```python
from build123d import *

# Parameters (mm, degrees)
F0_W     = 42
F0_H     = 22
F1_DEPTH = 13
F2_W     = 42
F2_H     = 22
F3_DEPTH = 5
F4_R     = 1
F5_DEPTH = 6
F6_R     = 5


with BuildPart() as f1:
    # F0 (on Top) → F1 (new body)
    with BuildSketch(Plane.XY):
        Rectangle(F0_W, F0_H)
        with BuildLine():
            ThreePointArc((-2.120368, -5.306732), (-19.5, 0), (-2.120368, 5.306732))
            Line((-2.120368, 5.306732), (2.120368, 5.306732))
            ThreePointArc((2.120368, 5.306732), (12.774302, 9.085882), (19.5, 0))
            ThreePointArc((19.5, 0), (12.774302, -9.085882), (2.120368, -5.306732))
            Line((2.120368, -5.306732), (-2.120368, -5.306732))
        make_face(mode=Mode.SUBTRACT)
    extrude(amount=F1_DEPTH)

    # F2 (on face) → F3 (join)
    with BuildSketch(Plane.XY.offset(13)):
        Rectangle(F2_W, F2_H)
    extrude(amount=F3_DEPTH)

    # F4 (on face) → F5 (cut)
    with BuildSketch(Plane.XY.offset(18)):
        with Locations((-4.52854, 0.924871)):
            Circle(F4_R)
        with Locations((4.52854, 0.924871)):
            Circle(F4_R)
    extrude(amount=-F5_DEPTH, mode=Mode.SUBTRACT)

    # F6
    f6_edges = [f1.edges().sort_by_distance(p)[0] for p in [
        (-21, -11, 9),
        (21, -11, 9),
        (-21, 11, 9),
        (21, 11, 9),
    ]]
    fillet(f6_edges, radius=F6_R)


solid = f1.part
```
Check sheet for the modelled part. Datum: model origin and axes. Units: mm. A direction names the side the tool comes from. Round coordinates to 2 decimals unless told otherwise and drop trailing zeros. Loops run counter-clockwise (first coordinate to the right, second up) from the corner with the lowest first, then second, coordinate; pieces in that order, holes last. Notation, with made-up numbers: (-34.75, 79) -> (-30.75, 79) arc R26 cw to (-30.75, 113) -> close; hole circle Ø9 at (4, 61). An arc over 180 degrees is marked (long way). Answer in a Markdown table with one row per item.
Q1. Release check for a two-part mould opening along X. For faces 1 (the face through (-3.991, 1.768, 15.535)), 2 (the face through (-20, 9, 9)), 3 (the face through (0, 11, 9)), 4 (the face through (21, 0, 9)) record: released by +X, released by -X, zero draft, split by the parting line, or undercut.
Data:
| item | result |
|---|---|
| face 1 | undercut |
| face 2 | released by -X |
| face 3 | zero draft |
| face 4 | released by +X |
Q2. Go/stop test with flat-tipped pins: P1, Ø5.5, axis at x = -2.5, y = -1.5, coming from the -Z side; P2, Ø1.6, axis at x = -4.53, y = 0.92, coming from the +Z side. Record where each tip stops, or that it passes through.
Data:
| item | result |
|---|---|
| P1 | stops at z = 13 |
| P2 | passes through |
Q3. Sectioned sample at B-B on z = 10. Enter the section's corners in (x, y).
Data:
| item | result |
|---|---|
| outline | (-21, -6) arc R5 ccw to (-16, -11) -> (16, -11) arc R5 ccw to (21, -6) -> (21, 6) arc R5 ccw to (16, 11) -> (-16, 11) arc R5 ccw to (-21, 6) -> close; hole (-2.12, -5.31) -> (2.12, -5.31) arc R9.5 ccw (long way) to (2.12, 5.31) -> (-2.12, 5.31) arc R9.5 ccw (long way) to start |
Q4. Sectioned sample at D-D on y = 7.5. Enter the section's corners in (x, z), then the cut area to 4 significant figures.
Data:
| item | result |
|---|---|
| outline | (-20.77, 0) -> (-15.83, 0) -> (-15.83, 13) -> (-4.17, 13) -> (-4.17, 0) -> (4.17, 0) -> (4.17, 13) -> (15.83, 13) -> (15.83, 0) -> (20.77, 0) -> (20.77, 18) -> (-20.77, 18) -> close |
| area | 444.5 mm^2 |
Q5. Thickness scan on L1, parallel to Y at x = -10, z = 6.25; L2, parallel to X at y = 1.5, z = 13.5; L3, parallel to Z at x = 12, y = 1.5. Record the ranges inside material, lowest first.
Data:
| item | result |
|---|---|
| L1 | y = -11 to -9.5, 9.5 to 11 |
| L2 | x = -21 to -5.35, -3.71 to 3.71, 5.35 to 21 |
| L3 | z = 13 to 18 |
Q6. Set-up check for faces 5 (the face through (0, 5.307, 6)), 6 (the face through (19, -10, 9)): record each of +Z, -Z, +X, -X, +Y, -Y from which the full face is reachable in a straight line by a thin tool's end or side.
Data:
| item | result |
|---|---|
| face 5 | -Z |
| face 6 | +Z, -Z, +X, -Y |
Q7. Sectioned sample at C-C on z = 15.75. Enter the section's corners in (x, y).
Data:
| item | result |
|---|---|
| outline | (-21, -6) arc R5 ccw to (-16, -11) -> (16, -11) arc R5 ccw to (21, -6) -> (21, 6) arc R5 ccw to (16, 11) -> (-16, 11) arc R5 ccw to (-21, 6) -> close; hole circle Ø2 at (-4.53, 0.92); hole circle Ø2 at (4.53, 0.92) |
Q8. Sectioned sample at A-A on x = -10. Enter the section's corners in (y, z).
Data:
| item | result |
|---|---|
| outline | (-11, 0) -> (-9.5, 0) -> (-9.5, 13) -> (9.5, 13) -> (9.5, 0) -> (11, 0) -> (11, 18) -> (-11, 18) -> close |
